```python
from build123d import *

# Parameters (mm, degrees)
SKETCH4_R           = 68.072
BOSS_EXTRUDE2_DEPTH = 1
SKETCH5_R           = 55.372
CUT_EXTRUDE5_DEPTH  = 2
SKETCH6_R           = 3.175
CUT_EXTRUDE6_DEPTH  = 2
CIRPATTERN1_COUNT   = 8
CUT_EXTRUDE11_DEPTH = 2


with BuildPart() as part:
    # Sketch4 → Boss-Extrude2 (new body)
    with BuildSketch(Plane.XY):
        Circle(SKETCH4_R)
    extrude(amount=BOSS_EXTRUDE2_DEPTH)

    # Sketch5 → Cut-Extrude5 (cut, through all)
    with BuildSketch(Plane.XY.offset(1)):
        Circle(SKETCH5_R)
    extrude(amount=-CUT_EXTRUDE5_DEPTH, mode=Mode.SUBTRACT)

    # Sketch6 → Cut-Extrude6 (cut, through all)
    with BuildSketch(Plane.XY.offset(1)):
        with Locations((61.722, 0)):
            Circle(SKETCH6_R)
    cut_extrude6 = extrude(amount=-CUT_EXTRUDE6_DEPTH, mode=Mode.SUBTRACT)

    # CirPattern1: Cut-Extrude6 ×8 about axis
    cirpattern1_axis = Axis((0, 0, 0), (0, 0, 1))
    for i in range(1, CIRPATTERN1_COUNT):
        add(cut_extrude6.rotate(cirpattern1_axis, i * 360 / CIRPATTERN1_COUNT), mode=Mode.SUBTRACT)

    # Sketch8 → Cut-Extrude11 (cut, through all)
    with BuildSketch(Plane.XY.offset(1)):
        Polygon((65.924300597, 28.681377492), (47.151068496, 20.905250146), (48.123084414, 18.558596133), (66.896316515, 26.334723479), align=None)
        Polygon((27.466357594, 62.990983081), (25.119703581, 63.962998999), (24.633695622, 62.789671993), (26.980349635, 61.817656075), align=None)
        Polygon((-25.119703581, 63.962998999), (-27.466357594, 62.990983081), (-26.980349635, 61.817656075), (-24.633695622, 62.789671993), align=None)
        Polygon((-62.990983081, 27.466357594), (-63.962998999, 25.119703581), (-62.789671993, 24.633695622), (-61.817656075, 26.980349635), align=None)
        Polygon((-63.962998999, -25.119703581), (-62.990983081, -27.466357594), (-61.817656075, -26.980349635), (-62.789671993, -24.633695622), align=None)
        Polygon((-27.466357594, -62.990983081), (-25.119703581, -63.962998999), (-24.633695622, -62.789671993), (-26.980349635, -61.817656075), align=None)
        Polygon((25.119703581, -63.962998999), (27.466357594, -62.990983081), (26.980349635, -61.817656075), (24.633695622, -62.789671993), align=None)
        Polygon((62.990983081, -27.466357594), (63.962998999, -25.119703581), (62.789671993, -24.633695622), (61.817656075, -26.980349635), align=None)
    extrude(amount=-CUT_EXTRUDE11_DEPTH, mode=Mode.SUBTRACT)


solid = part.part
```
Source: CAD feature listing. Evaluate the final solid. Frame: model axes, mm. A direction names the side the tool comes from. Round coordinates to 2 decimals unless told otherwise and drop trailing zeros. Loops run counter-clockwise (first coordinate to the right, second up) from the corner with the lowest first, then second, coordinate; pieces in that order, holes last. Notation, with made-up numbers: M -23,80 L 7,80 A15 cw 7,106 Z; hole C 1.5,-28.75 d6. An arc over 180 degrees is marked long. Use a Markdown table: item, result. Add a question column.
1. Cut plane D-D, the plane x = 31. Output: boundary loops of the cut face in (y, z).
2. Set-up query: faces 4 (the cylindrical face through (-0.36, -68.07, 0.49)), 5 (the flat face through (57.4, 22.4, 0.5)). Return all of +Z, -Z, +X, -X, +Y, -Y with unobstructed straight access to the full face (end or side cutting, diameter ignored); none if empty.
3. Ray query, line 1 along X through (y, z) = (9.5, 0.9); line 2 along Y through (x, z) = (55.5, 0.5); line 3 along X through (y, z) = (4, 0.7). Return the intervals inside material, ascending. Write a range as [from, to].
4. Cut plane C-C, the plane y = 14. Output: boundary loops of the cut face in (x, z), and give its area (3 significant figures).
5. Cut plane A-A, the plane x = 0. Output: boundary loops of the cut face in (y, z).
6. Contact query for a flat-ended pin moving along its axis: pin 1 (5 mm diameter, centred on x = 61.722, y = 0, fed in from -Z). Output: stop coordinate, or through.
7. Pull-direction query (Y, two-part tool) for faces 1 (the cylindrical face through (-44.858, 46.578, 0.507)), 2 (the flat face through (-5, 56, 1)), 3 (the cylindrical face through (47.881, -48.386, 0.493)); classes: +Y half, -Y half, draft (parallel to the pull), parting line (faces both ways), or undercut.
Solution:
| question | item | result |
|---|---|---|
| 1 | outline | M -60.6,0 L -45.88,0 L -45.88,1 L -60.6,1 Z; M 45.88,0 L 60.6,0 L 60.6,1 L 45.88,1 Z |
| 2 | face 4 | +Z, -Z, -Y |
| 2 | face 5 | +Z, -Z |
| 3 | line 1 | x = [-67.41, -54.55], [54.55, 67.41] |
| 3 | line 2 | y = [-39.42, 21.61], [24.36, 39.42] |
| 3 | line 3 | x = [-67.95, -55.23], [55.23, 67.95] |
| 4 | outline | M -66.62,0 L -53.57,0 L -53.57,1 L -66.62,1 Z; M 53.57,0 L 66.62,0 L 66.62,1 L 53.57,1 Z |
| 4 | area | 26.1 mm2 |
| 5 | outline | M -68.07,0 L -64.9,0 L -64.9,1 L -68.07,1 Z; M -58.55,0 L -55.37,0 L -55.37,1 L -58.55,1 Z; M 55.37,0 L 58.55,0 L 58.55,1 L 55.37,1 Z; M 64.9,0 L 68.07,0 L 68.07,1 L 64.9,1 Z |
| 6 | pin 1 | passes through |
| 7 | face 1 | undercut |
| 7 | face 2 | draft |
| 7 | face 3 | -Y half |
